Check sheet for the drawn part. Datum: minimum x, y, z corner. Units: mm. Give positions to 0.01 mm unless a question says otherwise; leave off trailing zeros. Order: outer loops, then holes, each group sorted by start corner. A loop starts at its lowest first (then second) coordinate and runs counter-clockwise, first axis right, second up. Notation, with made-up numbers: M 12,-3.75 L 62,-3.75 A10 ccw 62,11.25 Z; hole C -4.5,16.5 d1. An arc over 180 degrees is marked long. Answer in a Markdown table with one row per item. Add a question column.
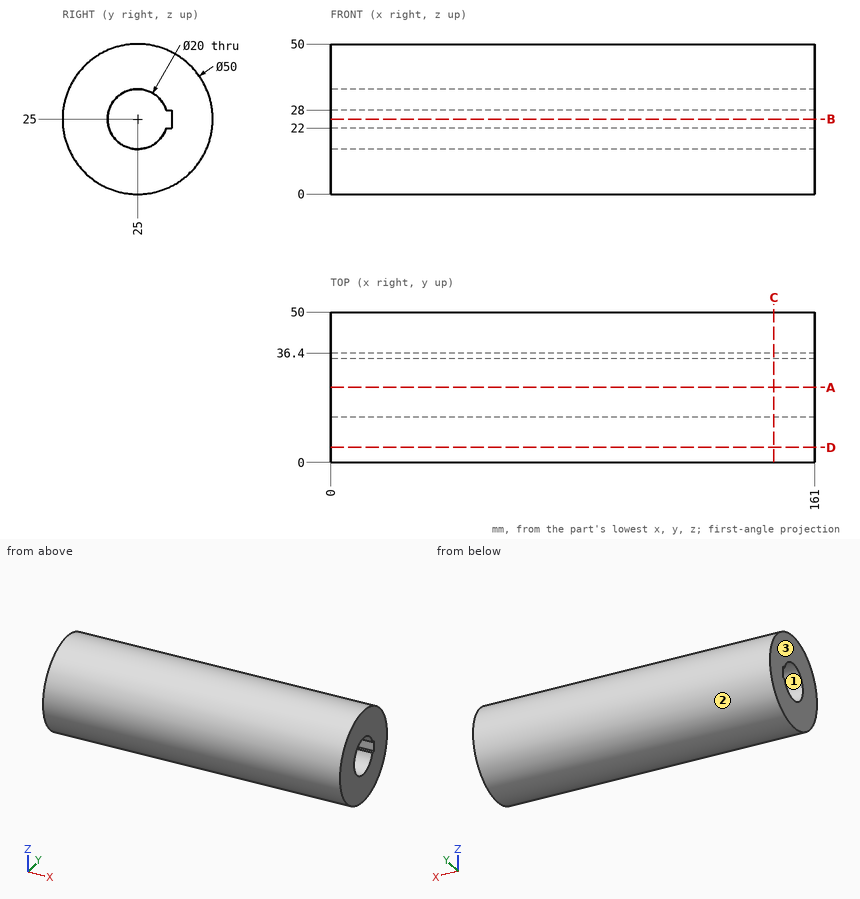
Q1. Go/stop test with flat-tipped pins: pin 1 (5 mm diameter, centred on x = 76.5, y = 39.5, fed in from +Z); pin 2 (8 mm diameter, centred on x = 93, z = 40.5, fed in from -Y); pin 3 (23 mm diameter, centred on y = 25, z = 25, fed in from -X); pin 4 (12 mm diameter, centred on x = 30, z = 18, fed in from +Y). Record where each tip stops, or that it passes through.
Q2. Cross-section at D-D (y = 5). Record the boundary of the cut face in (x, z), and give its area (3 significant figures).
Q3. Cross-section at C-C (x = 147.5). Record the boundary of the cut face in (y, z).
Q4. Cross-section at A-A (y = 25). Record the boundary of the cut face in (x, z).
Q5. Thickness scan on probe 1 along Y at (x, z) = (57.5, 25); probe 2 along Y at (x, z) = (85, 20); probe 3 along Z at (x, y) = (50.5, 36). Record the ranges inside material, lowest first.
Q6. Cross-section at B-B (z = 25). Record the boundary of the cut face in (x, y), and give its area (3 significant figures).
Q7. Draft check along Z on the marked faces 1, 2 and 3. Enter one of: pulls with the +Z half, pulls with the -Z half, needs draft (parallel to the pull), parting line crosses it, or undercut.
Values follow:
| question | item | result |
|---|---|---|
| 1 | pin 1 | z = 46.93 |
| 1 | pin 2 | y = 2.8 |
| 1 | pin 3 | x = 0 |
| 1 | pin 4 | y = 49.98 |
| 2 | outline | M 0,10 L 161,10 L 161,40 L 0,40 Z |
| 2 | area | 4,830 mm² |
| 3 | outline | C 25,25 d50; hole M 34.54,22 L 36.4,22 L 36.4,28 L 34.54,28 A10 ccw long Z |
| 4 | outline | M 0,0 L 161,0 L 161,15 L 0,15 Z; M 0,35 L 161,35 L 161,50 L 0,50 Z |
| 5 | probe 1 | 0 to 15, 36.4 to 50 |
| 5 | probe 2 | 0.51 to 16.34, 33.66 to 49.49 |
| 5 | probe 3 | 2.55 to 22, 28 to 47.45 |
| 6 | outline | M 0,0 L 161,0 L 161,15 L 0,15 Z; M 0,36.4 L 161,36.4 L 161,50 L 0,50 Z |
| 6 | area | 4,600 mm² |
| 7 | face 1 | undercut |
| 7 | face 2 | parting line crosses it |
| 7 | face 3 | needs draft |
